Build history of the part. All positions in model axes, mm. A direction names the side the tool comes from. Give positions to 0.01 mm unless a question says otherwise; leave off trailing zeros. Order: outer loops, then holes, each group sorted by start corner. A loop starts at its lowest first (then second) coordinate and runs counter-clockwise, first axis right, second up. Notation, with made-up numbers: (88, 66) - (109, 66) arc R23 cw to (109, 104) - close; hole circle Ø4 at (22.5, 23.5). An arc over 180 degrees is marked (long way). Use a Markdown table: item, result. Add a question column.
(1) Which spindle directions (+Z, -Z, +X, -X, +Y, -Y) get a long thin tool onto all of the face, cutting with end or side? Do faces 1 (the face through (-8.206, 11.375, -0.278)), 2 (the face through (-11.16, 1.32, -0.26)), 3 (the face through (7.395, -1.25, -0.264)), 4 (the face through (-9.81, -11.14, -0.26)), 5 (the face through (8.42, -1.15, -0.26)). Say none if no direction does.
(2) Mould opens along Y. For faces 6 (the face through (-11.178, 11.787, -0.278)), 7 (the face through (-12, 12.6, -1.25)), 8 (the face through (-11.97, 13.11, -0.26)), 9 (the face through (-7.76, 12.04, -0.26)) say: +Y half, -Y half, draft (parallel to the pull), parting line (faces both ways), or undercut.
(3) Slice it at D-D (x = -10). Write the cut outline in (y, z).
(4) Wall check: line 1 (X direction, y = 1.25, z = -1.2); line 2 (X direction, y = 2.25, z = -0.1); line 3 (Y direction, x = 5.5, z = -0.25). Give the ranges that are in metal, low to high.
(5) Flat gauge pins, fed straight in: pin 1 (3 mm diameter, centred on x = -8.5, y = 3.5, fed in from +Z); pin 2 (2 mm diameter, centred on y = 4, z = -0.5, fed in from -X); pin 3 (6.5 mm diameter, centred on x = -4.5, y = 3, fed in from +Z); pin 4 (1.4 mm diameter, centred on x = -11.5, y = 12.5, fed in from -Z). Where does each tip first touch, or does it go through?
(6) Slice it at C-C (z = -1.85). Write the cut outline in (x, y), then the cut area to 3 significant figures.
(7) Slice it at A-A (y = 0). Write the cut outline in (x, z).
(8) Slice it at B-B (x = 3.75). Write the cut outline in (y, z).
from build123d import *

# Parameters (mm, degrees)
BOSS_EXTRUDE1_START      = -1.25
BOSS_EXTRUDE1_DEPTH      = 2
BOSS_EXTRUDE2_DEPTH      = 1
BOSS_EXTRUDE2_DEPTH_BACK = 3
SKETCH3_W                = 2
SKETCH3_H                = 1
BOSS_EXTRUDE3_DEPTH      = 2


with BuildPart() as part:
    # Sketch1 → Boss-Extrude1 (new body)
    with BuildSketch(Plane.XY.offset(BOSS_EXTRUDE1_START)):
        with BuildLine():
            Line((2.436539132, -8.143296449), (-7.548366257, -11.130859638))
            ThreePointArc((-7.548366257, -11.130859638), (-9.842130636, -11.130694708), (-11.758669759, -9.870443602))
            ThreePointArc((-11.758669759, -9.870443602), (-11.965894787, -9.618177235), (-12.167708806, -9.361561504))
            ThreePointArc((-12.167708806, -9.361561504), (-12.519382992, -8.640760337), (-12.559604102, -7.839753896))
            Line((-12.559604102, -7.839753896), (-9.643676177, 11.234095698))
            ThreePointArc((-9.643676177, 11.234095698), (-9.365976364, 11.986499758), (-8.815011776, 12.569309399))
            ThreePointArc((-8.815011776, 12.569309399), (-8.54574672, 12.753908592), (-8.272617255, 12.932740434))
            ThreePointArc((-8.272617255, 12.932740434), (-6.067091304, 13.562827996), (-3.87804418, 12.877680022))
            Line((-3.87804418, 12.877680022), (4.758214838, 7.043393469))
            ThreePointArc((4.758214838, 7.043393469), (8.402381141, -1.284519818), (2.436539132, -8.143296449))
        make_face()
        with BuildLine():
            Line((-7.257137668, -9.99991839), (2.149887469, -7.185261573))
            ThreePointArc((2.149887469, -7.185261573), (7.413865713, -1.133399839), (4.198424857, 6.214758943))
            Line((4.198424857, 6.214758943), (-3.938007339, 11.711383912))
            ThreePointArc((-3.938007339, 11.711383912), (-5.571798261, 12.3507715), (-7.322050422, 12.229500574))
            ThreePointArc((-7.322050422, 12.229500574), (-8.258340754, 11.626081421), (-8.726639699, 10.615413149))
            Line((-8.726639699, 10.615413149), (-11.499609723, -7.523311304))
            ThreePointArc((-11.499609723, -7.523311304), (-11.354656305, -8.627730955), (-10.641413415, -9.483323638))
            ThreePointArc((-10.641413415, -9.483323638), (-9.007335115, -10.12197642), (-7.257137668, -9.99991839))
        make_face(mode=Mode.SUBTRACT)
    extrude(amount=BOSS_EXTRUDE1_DEPTH)

    # Sketch2 → Boss-Extrude2 (add, two sides: drawn at the far end of the back side and taken through both)
    with BuildSketch(Plane.XY.offset(0.75).offset(-BOSS_EXTRUDE2_DEPTH_BACK)):
        Polygon((-8.334933677, 10.530761514), (-11.300479962, 10.98412145), (-10.847120026, 13.949667735), (-7.881573741, 13.4963078), align=None)
    extrude(amount=BOSS_EXTRUDE2_DEPTH + BOSS_EXTRUDE2_DEPTH_BACK)

    # Sketch3 → Boss-Extrude3 (add)
    with BuildSketch(Plane(origin=(-12.683264825, 1.938962867, 0), x_dir=(0, 0, 1), z_dir=(-0.9885154283423572, 0.15111997859027873, 0))):
        with Locations((-0.25, 10.65024523)):
            Rectangle(SKETCH3_W, SKETCH3_H)
    extrude(amount=BOSS_EXTRUDE3_DEPTH)


solid = part.part
Solution:
| question | item | result |
|---|---|---|
| 1 | face 1 | none |
| 1 | face 2 | +Z, -Z, -X |
| 1 | face 3 | +Z, -Z |
| 1 | face 4 | +Z, -Z, -Y |
| 1 | face 5 | +Z, -Z, +X |
| 2 | face 6 | undercut |
| 2 | face 7 | draft |
| 2 | face 8 | +Y half |
| 2 | face 9 | undercut |
| 3 | outline | (-11.08, -1.25) - (-9.84, -1.25) - (-9.84, 0.75) - (-11.08, 0.75) - close; (2.29, -1.25) - (8.9, -1.25) - (8.9, 0.75) - (2.29, 0.75) - close; (10.79, -2.25) - (13.82, -2.25) - (13.82, 1.75) - (10.79, 1.75) - close |
| 4 | line 1 | -11.17 to -10.16, 7.4 to 8.41 |
| 4 | line 2 | -11.02 to -10.01, 7.15 to 8.2 |
| 4 | line 3 | -6.48 to -5.1, 5.1 to 6.48 |
| 5 | pin 1 | z = 0.75 |
| 5 | pin 2 | x = -10.9 |
| 5 | pin 3 | through |
| 5 | pin 4 | z = -2.25 |
| 6 | outline | (-11.3, 10.98) - (-8.33, 10.53) - (-7.88, 13.5) - (-10.85, 13.95) - close |
| 6 | area | 9.00 mm2 |
| 7 | outline | (-11.36, -1.25) - (-10.35, -1.25) - (-10.35, 0.75) - (-11.36, 0.75) - close; (7.5, -1.25) - (8.5, -1.25) - (8.5, 0.75) - (7.5, 0.75) - close |
| 8 | outline | (-7.63, -1.25) - (-6.5, -1.25) - (-6.5, 0.75) - (-7.63, 0.75) - close; (6.52, -1.25) - (7.72, -1.25) - (7.72, 0.75) - (6.52, 0.75) - close |
